Part model, mm, in its own coordinate system. A direction names the side the tool comes from. Give positions to 0.01 mm unless a question says otherwise; leave off trailing zeros. Write each loop counter-clockwise with the first axis right and the second up, starting at its lowest first coordinate (ties: lowest second). Pieces come first, ordered by that corner, then holes. Notation, with made-up numbers: M -9.5,-14 L 2.5,-14 A21 ccw 2.5,7 Z; hole C 79,-1 d9. An arc over 180 degrees is marked long. Use a Markdown table: item, result.
```python
from build123d import *

# Parameters (mm, degrees)
BOSS_EXTRUDE1_DEPTH = 4


with BuildPart() as part:
    # Sketch1 → Boss-Extrude1 (new body)
    with BuildSketch(Plane.XY):
        Polygon((162, 0), (0, 0), (0, -40), (71, -40), (71, -36), (91, -36), (91, -40), (162, -40), align=None)
        with BuildLine():
            ThreePointArc((8.5, -15), (10, -13.5), (11.5, -15))
            Line((11.5, -15), (11.5, -25))
            ThreePointArc((11.5, -25), (10, -26.5), (8.5, -25))
            Line((8.5, -25), (8.5, -15))
        make_face(mode=Mode.SUBTRACT)
        with BuildLine():
            Line((18.5, -25), (18.5, -15))
            ThreePointArc((18.5, -15), (20, -13.5), (21.5, -15))
            Line((21.5, -15), (21.5, -25))
            ThreePointArc((21.5, -25), (20, -26.5), (18.5, -25))
        make_face(mode=Mode.SUBTRACT)
        with BuildLine():
            ThreePointArc((28.5, -15), (30, -13.5), (31.5, -15))
            Line((31.5, -15), (31.5, -25))
            ThreePointArc((31.5, -25), (30, -26.5), (28.5, -25))
            Line((28.5, -25), (28.5, -15))
        make_face(mode=Mode.SUBTRACT)
        with BuildLine():
            Line((38.5, -25), (38.5, -15))
            ThreePointArc((38.5, -15), (40, -13.5), (41.5, -15))
            Line((41.5, -15), (41.5, -25))
            ThreePointArc((41.5, -25), (40, -26.5), (38.5, -25))
        make_face(mode=Mode.SUBTRACT)
        with BuildLine():
            ThreePointArc((68.5, -15), (70, -13.5), (71.5, -15))
            Line((71.5, -15), (71.5, -25))
            ThreePointArc((71.5, -25), (70, -26.5), (68.5, -25))
            Line((68.5, -25), (68.5, -15))
        make_face(mode=Mode.SUBTRACT)
        with BuildLine():
            Line((78.5, -25), (78.5, -15))
            ThreePointArc((78.5, -15), (80, -13.5), (81.5, -15))
            Line((81.5, -15), (81.5, -25))
            ThreePointArc((81.5, -25), (80, -26.5), (78.5, -25))
        make_face(mode=Mode.SUBTRACT)
        with BuildLine():
            Line((90.5, -25), (90.5, -15))
            ThreePointArc((90.5, -15), (92, -13.5), (93.5, -15))
            Line((93.5, -15), (93.5, -25))
            ThreePointArc((93.5, -25), (92, -26.5), (90.5, -25))
        make_face(mode=Mode.SUBTRACT)
        with BuildLine():
            ThreePointArc((100.5, -15), (102, -13.5), (103.5, -15))
            Line((103.5, -15), (103.5, -25))
            ThreePointArc((103.5, -25), (102, -26.5), (100.5, -25))
            Line((100.5, -25), (100.5, -15))
        make_face(mode=Mode.SUBTRACT)
        with BuildLine():
            ThreePointArc((120.5, -15), (122, -13.5), (123.5, -15))
            Line((123.5, -15), (123.5, -25))
            ThreePointArc((123.5, -25), (122, -26.5), (120.5, -25))
            Line((120.5, -25), (120.5, -15))
        make_face(mode=Mode.SUBTRACT)
        with BuildLine():
            Line((130.5, -25), (130.5, -15))
            ThreePointArc((130.5, -15), (132, -13.5), (133.5, -15))
            Line((133.5, -15), (133.5, -25))
            ThreePointArc((133.5, -25), (132, -26.5), (130.5, -25))
        make_face(mode=Mode.SUBTRACT)
        with BuildLine():
            ThreePointArc((140.5, -15), (142, -13.5), (143.5, -15))
            Line((143.5, -15), (143.5, -25))
            ThreePointArc((143.5, -25), (142, -26.5), (140.5, -25))
            Line((140.5, -25), (140.5, -15))
        make_face(mode=Mode.SUBTRACT)
        with BuildLine():
            Line((150.5, -25), (150.5, -15))
            ThreePointArc((150.5, -15), (152, -13.5), (153.5, -15))
            Line((153.5, -15), (153.5, -25))
            ThreePointArc((153.5, -25), (152, -26.5), (150.5, -25))
        make_face(mode=Mode.SUBTRACT)
        with BuildLine():
            ThreePointArc((48.5, -15), (50, -13.5), (51.5, -15))
            Line((51.5, -15), (51.5, -25))
            ThreePointArc((51.5, -25), (50, -26.5), (48.5, -25))
            Line((48.5, -25), (48.5, -15))
        make_face(mode=Mode.SUBTRACT)
        with BuildLine():
            Line((58.5, -25), (58.5, -15))
            ThreePointArc((58.5, -15), (60, -13.5), (61.5, -15))
            Line((61.5, -15), (61.5, -25))
            ThreePointArc((61.5, -25), (60, -26.5), (58.5, -25))
        make_face(mode=Mode.SUBTRACT)
        with BuildLine():
            Line((110.5, -25), (110.5, -15))
            ThreePointArc((110.5, -15), (112, -13.5), (113.5, -15))
            Line((113.5, -15), (113.5, -25))
            ThreePointArc((113.5, -25), (112, -26.5), (110.5, -25))
        make_face(mode=Mode.SUBTRACT)
    extrude(amount=BOSS_EXTRUDE1_DEPTH)


solid = part.part
```
1. Drop a flat-ended pin along its axis: P1, Ø2, axis at y = -18, z = 1, coming from the -X side. Give the stop position or say it passes through.
Findings below:
| item | result |
|---|---|
| P1 | x = 0 |
2. Tool access for faces 1 (the flat face through (0, -20, 2)), 2 (the flat face through (140.5, -20, 2)): list every direction of +Z, -Z, +X, -X, +Y, -Y with a clear straight run to the whole face (end or side of a thin tool).
Findings below:
| item | result |
|---|---|
| face 1 | +Z, -Z, -X, +Y, -Y |
| face 2 | +Z, -Z |
3. Drill centre lines: L1, parallel to X at y = -38, z = 3.2; L2, parallel to Y at x = 84, z = 1.5; L3, parallel to Y at x = 79, z = 1.55. Where is each one in solid material? Low to high.
Findings below:
| item | result |
|---|---|
| L1 | 0 to 71, 91 to 162 |
| L2 | -36 to 0 |
| L3 | -36 to -26.12, -13.88 to 0 |
4. Cut at C-C, the plane x = 152. Give the cut face in (y, z).
Findings below:
| item | result |
|---|---|
| outline | M -40,0 L -26.5,0 L -26.5,4 L -40,4 Z; M -13.5,0 L 0,0 L 0,4 L -13.5,4 Z |
5. Cut at B-B, the plane y = -22. State how many separate pieces and enclosed holes the cut face has, then the cut area to 3 significant figures.
Findings below:
| item | result |
|---|---|
| separate pieces | 16 |
| enclosed holes | 0 |
| area | 468 mm2 |
6. Two-plate mould, pull along Y, no slides. Class faces 3 (the flat face through (82, 0, 2)), 4 (the cylindrical face through (132, -13.5, 2)), 5 (the flat face through (35, -40, 2)), 6 (the cylindrical face through (20, -13.5, 2)): released by +Y, released by -Y, zero draft, split by the parting line, or undercut.
Findings below:
| item | result |
|---|---|
| face 3 | released by +Y |
| face 4 | undercut |
| face 5 | released by -Y |
| face 6 | undercut |
7. Cut at A-A, the plane x = 80. Give the cut face in (y, z).
Findings below:
| item | result |
|---|---|
| outline | M -36,0 L -26.5,0 L -26.5,4 L -36,4 Z; M -13.5,0 L 0,0 L 0,4 L -13.5,4 Z |
